from build123d import *

# Parameters (mm, degrees)
SKETCH3_W             = 140.131000148
SKETCH3_H             = 140
BOSS_EXTRUDE3_DEPTH   = 10
SKETCH3_7_OUTSIDE_W   = 181.797
SKETCH3_7_OUTSIDE_H   = 181.666
SKETCH3_7_OUTSIDE_W_2 = 140.131000148
SKETCH3_7_OUTSIDE_H_2 = 140
SKETCH3_7_OUTSIDE_R   = 33.499999497
CUT_EXTRUDE5_DEPTH    = 10
SKETCH2_R             = 2.25
CUT_EXTRUDE6_DEPTH    = 10


with BuildPart() as part:
    # Sketch3 → Boss-Extrude3 (new body)
    with BuildSketch(Plane.XY):
        with Locations((-121.856065437, 0)):
            Rectangle(SKETCH3_W, SKETCH3_H)
    extrude(amount=BOSS_EXTRUDE3_DEPTH)

    # Sketch3<7> outside → Cut-Extrude5 (cut)
    # profile 1 of 2: a face of its own
    with BuildSketch(Plane.XY):
        with Locations((-121.8565, 0)):
            Rectangle(SKETCH3_7_OUTSIDE_W, SKETCH3_7_OUTSIDE_H)
        with Locations((-121.856065437, 0)):
            Rectangle(SKETCH3_7_OUTSIDE_W_2, SKETCH3_7_OUTSIDE_H_2, mode=Mode.SUBTRACT)
    # profile 2 of 2: a face of its own
    with BuildSketch(Plane.XY):
        with Locations((-121.856065437, 0)):
            Circle(SKETCH3_7_OUTSIDE_R)
    extrude(amount=CUT_EXTRUDE5_DEPTH, mode=Mode.SUBTRACT)

    # Sketch2 → Cut-Extrude6 (cut)
    with BuildSketch(Plane.XY):
        with Locations((-107.548664291, 34.645482469)):
            Circle(SKETCH2_R)
        with Locations((-95.38278871, 26.516504294)):
            Circle(SKETCH2_R)
        with Locations((-87.253810535, 14.350628714)):
            Circle(SKETCH2_R)
        with Locations((-84.399293004, 0)):
            Circle(SKETCH2_R)
        with Locations((-87.253810535, -14.350628714)):
            Circle(SKETCH2_R)
        with Locations((-95.38278871, -26.516504294)):
            Circle(SKETCH2_R)
        with Locations((-107.548664291, -34.645482469)):
            Circle(SKETCH2_R)
        with Locations((-121.899293004, -37.5)):
            Circle(SKETCH2_R)
        with Locations((-136.249921718, -34.645482469)):
            Circle(SKETCH2_R)
        with Locations((-148.415797299, -26.516504294)):
            Circle(SKETCH2_R)
        with Locations((-156.544775474, -14.350628714)):
            Circle(SKETCH2_R)
        with Locations((-159.399293004, 0)):
            Circle(SKETCH2_R)
        with Locations((-156.544775474, 14.350628714)):
            Circle(SKETCH2_R)
        with Locations((-148.415797299, 26.516504294)):
            Circle(SKETCH2_R)
        with Locations((-136.249921718, 34.645482469)):
            Circle(SKETCH2_R)
        with Locations((-121.899293004, 37.5)):
            Circle(SKETCH2_R)
    extrude(amount=CUT_EXTRUDE6_DEPTH, mode=Mode.SUBTRACT)


solid = part.part
Verification items for the finished model (mm, model axes). Coordinates: 2 decimals unless noted, no trailing zeros. Write each loop counter-clockwise with the first axis right and the second up, starting at its lowest first coordinate (ties: lowest second). Pieces come first, ordered by that corner, then holes. Notation, with made-up numbers: M 44,85.5 L 58,85.5 A28 cw 58,112.5 Z; hole C -10.75,-23 d1. An arc over 180 degrees is marked long. Use a Markdown table: item, result.
Q1. Go/stop test with flat-tipped pins: P1, Ø4, axis at x = -156.54, y = 14.35, coming from the -Z side; P2, Ø7, axis at x = -87.25, y = -14.35, coming from the -Z side. Record where each tip stops, or that it passes through.
Reply:
| item | result |
|---|---|
| P1 | passes through |
| P2 | stops at z = 0 |
Q2. Sectioned sample at B-B, the plane x = -113. Record the boundary of the cut face in (y, z), plus the area to 3 significant figures.
Reply:
| item | result |
|---|---|
| outline | M -70,0 L -32.31,0 L -32.31,10 L -70,10 Z; M 32.31,0 L 70,0 L 70,10 L 32.31,10 Z |
| area | 754 mm² |
Q3. Sectioned sample at A-A, the plane y = 0. Record the boundary of the cut face in (x, z), plus the area to 3 significant figures.
Reply:
| item | result |
|---|---|
| outline | M -191.92,0 L -161.65,0 L -161.65,10 L -191.92,10 Z; M -157.15,0 L -155.36,0 L -155.36,10 L -157.15,10 Z; M -88.36,0 L -86.65,0 L -86.65,10 L -88.36,10 Z; M -82.15,0 L -51.79,0 L -51.79,10 L -82.15,10 Z |
| area | 641 mm² |
Q4. Draft check along X on faces 1 (the face through (-147.378, -28.513, 4.93)), 2 (the face through (-191.922, -1, 5)), 3 (the face through (-123, -70, 5)). Enter one of: +X half, -X half, draft (parallel to the pull), parting line (faces both ways), or undercut.
Reply:
| item | result |
|---|---|
| face 1 | undercut |
| face 2 | -X half |
| face 3 | draft |
Q5. Sectioned sample at C-C, the plane z = 1.75. Count the separate pieces of the cut face and the enclosed holes in it, plus the area to 3 significant figures.
Reply:
| item | result |
|---|---|
| separate pieces | 1 |
| enclosed holes | 17 |
| area | 15,800 mm² |
Q6. Thickness scan on line 1 (X direction, y = 24.5, z = 9); line 2 (X direction, y = 26, z = 3.5); line 3 (Y direction, x = -135.5, z = 8.5). Record the ranges inside material, lowest first.
Reply:
| item | result |
|---|---|
| line 1 | x = -191.92 to -149.41, -147.42 to -144.7, -99.01 to -96.38, -94.38 to -51.79 |
| line 2 | x = -191.92 to -150.61, -146.23 to -142.98, -100.73 to -97.57, -93.19 to -51.79 |
| line 3 | y = -70 to -36.77, -32.52 to -30.6, 30.6 to 32.52, 36.77 to 70 |
